Study the drawing (mm; zero at the part's minimum x, y, z) and answer. Round coordinates to 2 decimals unless told otherwise and drop trailing zeros. Loops run counter-clockwise (first coordinate to the right, second up) from the corner with the lowest first, then second, coordinate; pieces in that order, holes last. Notation, with made-up numbers: (58, -10) - (92, -10) arc R18 ccw to (92, 0) - close; hole circle Ø10 at (-2, -29.5). An arc over 180 degrees is marked (long way). One line per item, written item: value.
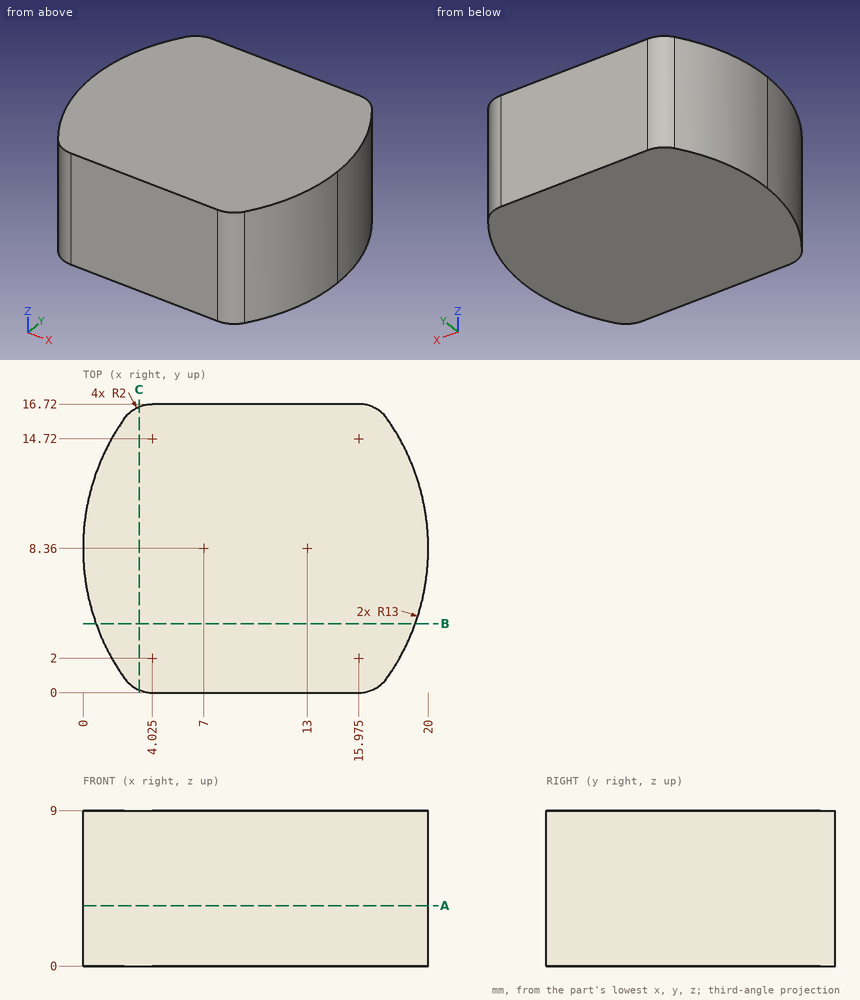
1) A cutting plane is placed at C-C on x = 3.25. Give the vertices of the cut face in (y, z).
Final values:
outline: (0.16, 0) - (16.56, 0) - (16.56, 9) - (0.16, 9) - close
2) A cutting plane is placed at B-B on y = 4. Give the vertices of the cut face in (x, z), and give its area (3 significant figures).
Final values:
outline: (0.75, 0) - (19.25, 0) - (19.25, 9) - (0.75, 9) - close
area: 166 mm2
3) Each of these flat-tipped pins is pushed along its axis until it touches: pin 1 Ø1.5 at (y, z) = (15, 3.5) entering from +X; pin 2 Ø3 at (y, z) = (12, 4.5) entering from -X; pin 3 Ø3 at (y, z) = (4, 3) entering from -X. Where does it stop, or does it pass through?
Final values:
pin 1: x = 18.59
pin 2: x = 0.18
pin 3: x = 0.32
4) A cutting plane is placed at A-A on z = 3.5. Give the vertices of the cut face in (x, y) (3 decimals), and give its area (3 significant figures).
Final values:
outline: (2.393, 0.844) arc R2 ccw to (4.025, 0) - (15.975, 0) arc R2 ccw to (17.607, 0.844) arc R13 ccw to (17.607, 15.876) arc R2 ccw to (15.975, 16.72) - (4.025, 16.72) arc R2 ccw to (2.393, 15.876) arc R13 ccw to start
area: 302 mm2
5) Consider L1, parallel to X at y = 16, z = 2.25; L2, parallel to X at y = 5, z = 7.75; L3, parallel to Y at x = 1.75, z = 0.5. Determine where each line is inside the solid, lowest interval first.
Final values:
L1: 2.49 to 17.51
L2: 0.44 to 19.56
L3: 1.85 to 14.87
